Here's the drawing with two shaded views (mm, measured from the low corner). I have some questions. Round coordinates to 2 decimals unless told otherwise and drop trailing zeros. Loops run counter-clockwise (first coordinate to the right, second up) from the corner with the lowest first, then second, coordinate; pieces in that order, holes last.
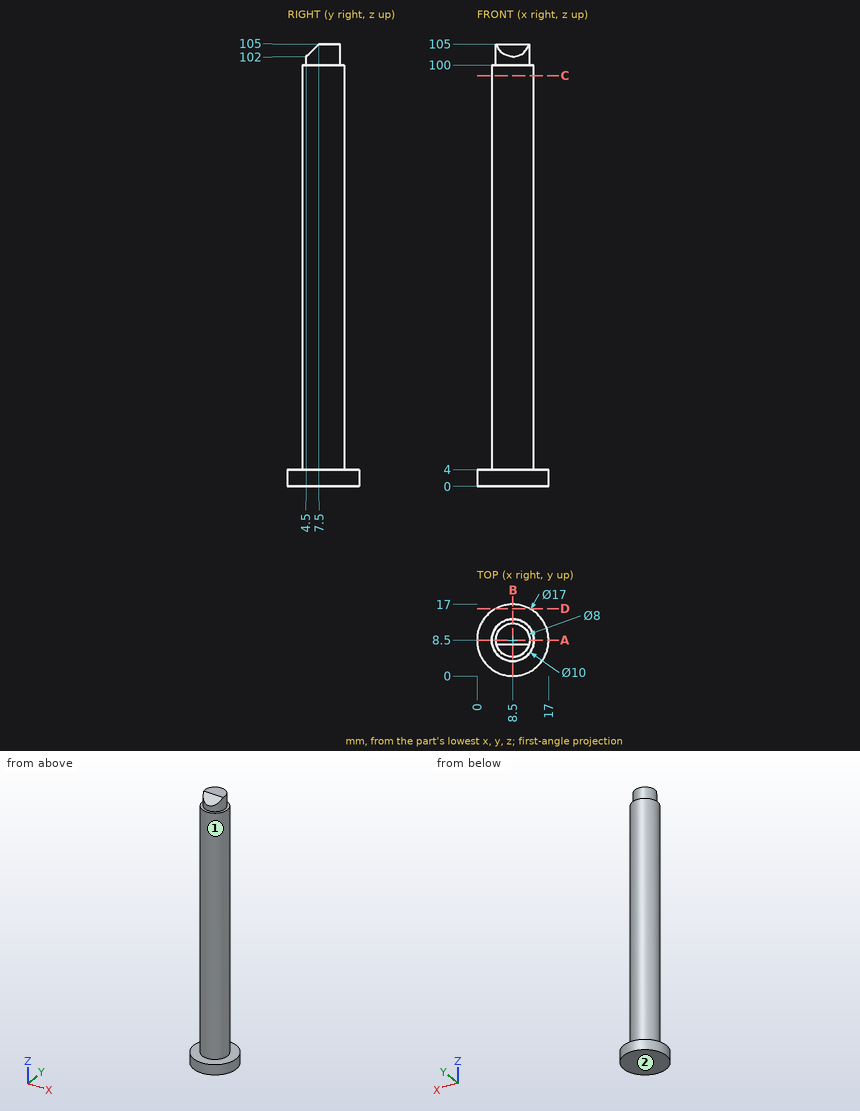
Item 1: If we section it at D-D, the plane y = 16: Please give me the cut outline in (x, z).
Results list:
outline: (4.5, 0) - (12.5, 0) - (12.5, 4) - (4.5, 4) - close
Item 2: If we section it at B-B, the plane x = 8.5: Please give me the cut outline in (y, z).
Results list:
outline: (0, 0) - (17, 0) - (17, 4) - (13.5, 4) - (13.5, 100) - (12.5, 100) - (12.5, 105) - (7.5, 105) - (4.5, 102) - (4.5, 100) - (3.5, 100) - (3.5, 4) - (0, 4) - close
Item 3: If I drill on line 1 along Z through (x, y) = (8.25, 15); line 2 along Z through (x, y) = (4, 9.25); line 3 along X through (y, z) = (5, 52), over which ranges is the centre line in solid material (lowest first)?
Results list:
line 1: z = 0 to 4
line 2: z = 0 to 100
line 3: x = 4.93 to 12.07
Item 4: Will these pins go through, and if not, where does the flat tip stop? pin 1 (3 mm diameter, centred on y = 3, z = 46, fed in from -X); pin 2 (3 mm diameter, centred on x = 5.5, z = 15, fed in from +Y); pin 3 (1 mm diameter, centred on x = 14, y = 2, fed in from +Z); pin 4 (5 mm diameter, centred on x = 8.5, y = 5.5, fed in from +Z).
Results list:
pin 1: stops at x = 5.5
pin 2: stops at y = 13.27
pin 3: stops at z = 4
pin 4: stops at z = 105
Item 5: If we section it at C-C, the plane z = 97.5: Please give me the cut outline in (x, y), then the cut area to 3 significant figures.
Results list:
outline: circle Ø10 at (8.5, 8.5)
area: 78.5 mm2
Item 6: We'd pull the mould along Y, two halves only. Please class the marked faces 1 and 2: released by +Y, released by -Y, zero draft, split by the parting line, or undercut.
Results list:
face 1: split by the parting line
face 2: zero draft
Item 7: If we section it at A-A, the plane y = 8.5: Please give me the cut outline in (x, z).
Results list:
outline: (0, 0) - (17, 0) - (17, 4) - (13.5, 4) - (13.5, 100) - (12.5, 100) - (12.5, 105) - (4.5, 105) - (4.5, 100) - (3.5, 100) - (3.5, 4) - (0, 4) - close
